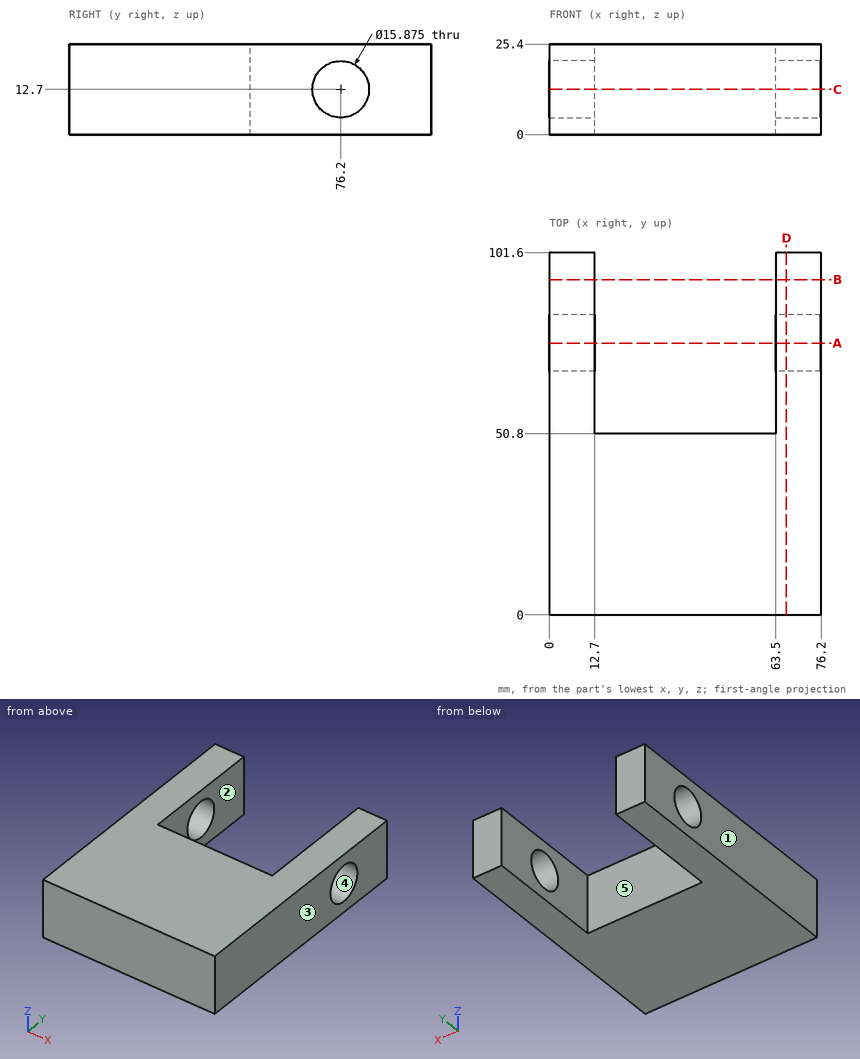
The drawing under review shows one solid part. Ordinate dimensions are in mm from its lowest x, y, z. A direction names the side the tool comes from. Give positions to 0.01 mm unless a question says otherwise; leave off trailing zeros. Loops run counter-clockwise (first coordinate to the right, second up) from the corner with the lowest first, then second, coordinate; pieces in that order, holes last. Notation, with made-up numbers: M 31.25,87.5 L 53.25,87.5 A23 cw 53.25,104.5 Z; hole C 45.25,16 d11. An arc over 180 degrees is marked long. Return JSON: item names as keys, results as strings. Group by question number.
Item 1: For probe 1 along Z at (x, y) = (3.25, 76.2); probe 2 along Y at (x, z) = (67.25, 12.7); probe 3 along X at (y, z) = (52, 12.75), list the stretches that pass through material, from the lowest coordinate up.
Item 2: Insertion check: pin 1 Ø12 at (x, z) = (41, 3.5) entering from +Y; pin 2 Ø6 at (x, z) = (27, 13) entering from -Y. Each pin has a flat end and moves straight along its axis. Give the tip position at first contact, or say it passes through.
Item 3: We need section A-A (y = 76.2). Give the boundary of the cut face in (x, z).
Item 4: We need section C-C (z = 12.7). Give the boundary of the cut face in (x, y).
Item 5: Mouldability with a two-part tool opening along X and no side actions: class the marked faces 3, 4 and 5 as released by +X, released by -X, zero draft, split by the parting line, or undercut.
Item 6: Tool access review of the marked faces 1 and 2: name each direction out of +Z, -Z, +X, -X, +Y, -Y from which nothing blocks a thin tool from reaching the whole face with its end or side.
Item 7: We need section D-D (x = 66.5). Give the boundary of the cut face in (y, z) (1 decimal), and give its area (3 significant figures).
Item 8: We need section B-B (y = 94). Give the boundary of the cut face in (x, z), and give its area (3 significant figures).
Output:
{
 "1": {"probe 1": "z = 0 to 4.76, 20.64 to 25.4", "probe 2": "y = 0 to 68.26, 84.14 to 101.6", "probe 3": "x = 0 to 12.7, 63.5 to 76.2"},
 "2": {"pin 1": "stops at y = 50.8", "pin 2": "stops at y = 0"},
 "3": {"outline": "M 0,0 L 12.7,0 L 12.7,4.76 L 0,4.76 Z; M 0,20.64 L 12.7,20.64 L 12.7,25.4 L 0,25.4 Z; M 63.5,0 L 76.2,0 L 76.2,4.76 L 63.5,4.76 Z; M 63.5,20.64 L 76.2,20.64 L 76.2,25.4 L 63.5,25.4 Z"},
 "4": {"outline": "M 0,0 L 76.2,0 L 76.2,68.26 L 63.5,68.26 L 63.5,50.8 L 12.7,50.8 L 12.7,68.26 L 0,68.26 Z; M 0,84.14 L 12.7,84.14 L 12.7,101.6 L 0,101.6 Z; M 63.5,84.14 L 76.2,84.14 L 76.2,101.6 L 63.5,101.6 Z"},
 "5": {"face 3": "released by +X", "face 4": "zero draft", "face 5": "undercut"},
 "6": {"face 1": "+Z, -Z, -X, +Y, -Y", "face 2": "+Z, -Z, +Y"},
 "7": {"outline": "M 0,0 L 101.6,0 L 101.6,25.4 L 0,25.4 Z; hole C 76.2,12.7 d15.9", "area": "2,380 mm^2"},
 "8": {"outline": "M 0,0 L 12.7,0 L 12.7,25.4 L 0,25.4 Z; M 63.5,0 L 76.2,0 L 76.2,25.4 L 63.5,25.4 Z", "area": "645 mm^2"}
}
